from build123d import *

# Parameters (mm, degrees)
SKETCH1_R           = 60.625
SKETCH1_R_2         = 45
BOSS_EXTRUDE1_DEPTH = 4
SKETCH2_R           = 49
SKETCH2_R_2         = 45
BOSS_EXTRUDE2_DEPTH = 52
SKETCH3_W           = 8
SKETCH3_H           = 38
SKETCH3_W_2         = 15
SKETCH3_H_2         = 8
BOSS_EXTRUDE3_DEPTH = 13
SKETCH4_R           = 1.3
CUT_EXTRUDE1_DEPTH  = 7.2
BOSS_EXTRUDE4_DEPTH = 4
SKETCH7_W           = 10
SKETCH7_H           = 24
CUT_EXTRUDE2_DEPTH  = 8
SKETCH8_R           = 5
CUT_EXTRUDE3_DEPTH  = 110.441337026
CUT_EXTRUDE4_REACH  = 104.405
SKETCH9_R           = 1.5


with BuildPart() as part:
    # Sketch1 → Boss-Extrude1 (new body)
    with BuildSketch(Plane(origin=(0, 0, 0), x_dir=(1, 0, 0), z_dir=(0, 1, 0))):
        with Locations(Location((0, 0, 0), (0, 0, 270))):
            Circle(SKETCH1_R)
        with Locations(Location((0, 0, 0), (0, 0, 270))):
            Circle(SKETCH1_R_2, mode=Mode.SUBTRACT)
    extrude(amount=BOSS_EXTRUDE1_DEPTH)

    # Sketch2 → Boss-Extrude2 (add)
    with BuildSketch(Plane(origin=(0, 4, 0), x_dir=(1, 0, 0), z_dir=(0, 1, 0))):
        with Locations(Location((0, 0, 0), (0, 0, 90))):
            Circle(SKETCH2_R)
        with Locations(Location((0, 0, 0), (0, 0, 270))):
            Circle(SKETCH2_R_2, mode=Mode.SUBTRACT)
    extrude(amount=BOSS_EXTRUDE2_DEPTH)

    # Sketch3 → Boss-Extrude3 (add, symmetric)
    with BuildSketch(Plane.XY):
        with Locations((15.25, 19)):
            Rectangle(SKETCH3_W, SKETCH3_H)
        with Locations((-39.25, 34)):
            Rectangle(SKETCH3_W_2, SKETCH3_H_2)
    extrude(amount=BOSS_EXTRUDE3_DEPTH, both=True)


with BuildPart() as boss_extrude3_piece_1:
    # of the separate pieces the step leaves, piece 1, a body of its own (boss_extrude3_pieces)
    add(part.part.solids().sort_by_distance((0, 0, 60.625))[0])


with BuildPart() as boss_extrude3_piece_2:
    # of the separate pieces the step leaves, piece 2, a body of its own (boss_extrude3_pieces)
    add(part.part.solids().sort_by_distance((11.25, 0, -13))[0])


with BuildPart() as cut_extrude1_tool:
    # Sketch4 → Cut-Extrude1 (new body)
    with BuildSketch(Plane(origin=(0, 38, 0), x_dir=(1, 0, 0), z_dir=(0, 1, 0))):
        with Locations(Location((13.75, 5, 0), (0, 0, 270))):
            Circle(SKETCH4_R)
        with Locations(Location((13.75, -5, 0), (0, 0, 270))):
            Circle(SKETCH4_R)
        with Locations(Location((-34.25, 5, 0), (0, 0, 270))):
            Circle(SKETCH4_R)
        with Locations(Location((-34.25, -5, 0), (0, 0, 270))):
            Circle(SKETCH4_R)
    extrude(amount=-CUT_EXTRUDE1_DEPTH)


with BuildPart() as boss_extrude3_piece_1_1:
    add(boss_extrude3_piece_1.part)

    # Cut-Extrude1: cut by cut_extrude1_tool
    add(cut_extrude1_tool.part, mode=Mode.SUBTRACT)



with BuildPart() as boss_extrude3_piece_2_1:
    add(boss_extrude3_piece_2.part)

    # Cut-Extrude1: cut by cut_extrude1_tool
    add(cut_extrude1_tool.part, mode=Mode.SUBTRACT)


with BuildPart() as boss_extrude3_piece_1_2:
    add(boss_extrude3_piece_1_1.part)

    add(boss_extrude3_piece_2_1.part)  # Boss-Extrude4 merges Boss-Extrude3 piece 2
    # Sketch5 → Boss-Extrude4 (add)
    with BuildSketch(Plane.XZ):
        with BuildLine():
            Line((11.25, 13), (25.249838503, 37.248431585))
            ThreePointArc((25.249838503, 37.248431585), (45, 0), (25.249838503, -37.248431585))
            Line((25.249838503, -37.248431585), (11.25, -13))
            Line((11.25, -13), (11.25, 13))
        make_face()
        with BuildLine():
            Line((24.25, -19.516660498), (27.361802413, -24.906460381))
            ThreePointArc((27.361802413, -24.906460381), (37, 0), (27.361802413, 24.906460381))
            Line((27.361802413, 24.906460381), (24.25, 19.516660498))
            Line((24.25, 19.516660498), (24.25, -19.516660498))
        make_face(mode=Mode.SUBTRACT)
    extrude(amount=-BOSS_EXTRUDE4_DEPTH)

    # Sketch7 → Cut-Extrude2 (cut)
    with BuildSketch(Plane.ZY.offset(-11.25)):
        with Locations((0, 17)):
            Rectangle(SKETCH7_W, SKETCH7_H)
    extrude(amount=-CUT_EXTRUDE2_DEPTH, mode=Mode.SUBTRACT)

    # Sketch8 → Cut-Extrude3 (cut, through all)
    with BuildSketch(Plane.ZY.offset(-11.25)):
        with Locations((0, 14)):
            Circle(SKETCH8_R)
    extrude(amount=-CUT_EXTRUDE3_DEPTH, mode=Mode.SUBTRACT)

    # Sketch9 → Cut-Extrude4 (cut, up to next)
    with BuildSketch(Plane.XZ, mode=Mode.PRIVATE) as cut_extrude4_sk1:
        with Locations(Location((54.5, 0, 0), (0, 0, 270))):
            Circle(SKETCH9_R)
    cut_extrude4_tool1 = extrude(cut_extrude4_sk1.sketch, amount=-CUT_EXTRUDE4_REACH, mode=Mode.PRIVATE) & boss_extrude3_piece_1_2.part
    # Sketch9 → Cut-Extrude4 (cut, up to next)
    with BuildSketch(Plane.XZ, mode=Mode.PRIVATE) as cut_extrude4_sk2:
        with Locations(Location((0, -54.5, 0), (0, 0, 270))):
            Circle(SKETCH9_R)
    cut_extrude4_tool2 = extrude(cut_extrude4_sk2.sketch, amount=-CUT_EXTRUDE4_REACH, mode=Mode.PRIVATE) & boss_extrude3_piece_1_2.part
    # Sketch9 → Cut-Extrude4 (cut, up to next)
    with BuildSketch(Plane.XZ, mode=Mode.PRIVATE) as cut_extrude4_sk3:
        with Locations(Location((-54.5, 0, 0), (0, 0, 270))):
            Circle(SKETCH9_R)
    cut_extrude4_tool3 = extrude(cut_extrude4_sk3.sketch, amount=-CUT_EXTRUDE4_REACH, mode=Mode.PRIVATE) & boss_extrude3_piece_1_2.part
    # Sketch9 → Cut-Extrude4 (cut, up to next)
    with BuildSketch(Plane.XZ, mode=Mode.PRIVATE) as cut_extrude4_sk4:
        with Locations(Location((0, 54.5, 0), (0, 0, 270))):
            Circle(SKETCH9_R)
    cut_extrude4_tool4 = extrude(cut_extrude4_sk4.sketch, amount=-CUT_EXTRUDE4_REACH, mode=Mode.PRIVATE) & boss_extrude3_piece_1_2.part
    add(cut_extrude4_tool1.solids().sort_by_distance((54.5, 0, 0))[0], mode=Mode.SUBTRACT)
    add(cut_extrude4_tool2.solids().sort_by_distance((0, 0, -54.5))[0], mode=Mode.SUBTRACT)
    add(cut_extrude4_tool3.solids().sort_by_distance((-54.5, 0, 0))[0], mode=Mode.SUBTRACT)
    add(cut_extrude4_tool4.solids().sort_by_distance((0, 0, 54.5))[0], mode=Mode.SUBTRACT)


solid = boss_extrude3_piece_1_2.part
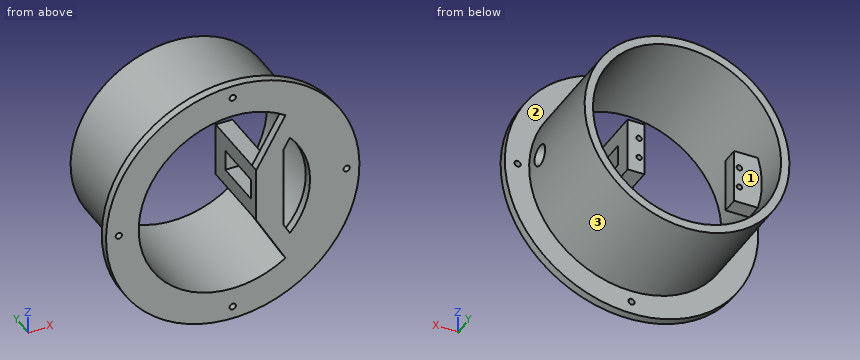
Here's how the part is built. I have some questions about the finished solid (model axes, mm). Face numbers are marked on the shaded views. Give positions to 0.01 mm unless a question says otherwise; leave off trailing zeros. Loops run counter-clockwise (first coordinate to the right, second up) from the corner with the lowest first, then second, coordinate; pieces in that order, holes last. Notation, with made-up numbers: (87.25, 24) -> (134.25, 24) arc R6 cw to (134.25, 30) -> close; hole circle Ø11 at (44.5, 13.25). An arc over 180 degrees is marked (long way). Answer as a JSON object with one key per item and string values. Group by question number.
Item 1: Imagine slicing it at B-B on x = 0. Write out the boundary of the cut face in (y, z) (3 decimals), then the cut area to 3 significant figures.
Item 2: I need wall thicknesses on L1, parallel to X at y = 29.5, z = -11.5; L2, parallel to X at y = 43, z = 0; L3, parallel to Y at x = 45.85, z = 0. Which ranges of each line are inside material? Lowest first, please.
Item 3: Will these pins go through, and if not, where does the flat tip stop? pin 1 (6.5 mm diameter, centred on x = 14, z = 1, fed in from +Y); pin 2 (2 mm diameter, centred on y = 1, z = -8.5, fed in from +X); pin 3 (6.5 mm diameter, centred on x = -39.5, y = 36, fed in from -Z); pin 4 (12 mm diameter, centred on x = 20, z = -14.5, fed in from -Y).
Item 4: Imagine slicing it at A-A on y = 26. Write out the boundary of the cut face in (x, z), then the cut area to 3 significant figures.
Item 5: Thinking about a two-plate mould opening in X: for the marked faces 1, 2 and 3, which applies, pulls with the +X half, pulls with the -X half, needs draft (parallel to the pull), parting line crosses it, or undercut?
Item 6: Imagine slicing it at C-C on z = 39.5. Write out the boundary of the cut face in (x, y), then the cut area to 3 significant figures.
Item 7: Imagine slicing it at D-D on x = 54.5. Write out the boundary of the cut face in (y, z).
Answer list:
{
 "1": {"outline": "(0, -60.625) -> (4, -60.625) -> (4, -56) -> (0, -56) -> close; (0, -53) -> (4, -53) -> (4, -49) -> (56, -49) -> (56, -45) -> (0, -45) -> close; (0, 45) -> (56, 45) -> (56, 49) -> (4, 49) -> (4, 53) -> (0, 53) -> close; (0, 56) -> (4, 56) -> (4, 60.625) -> (0, 60.625) -> close", "area": "517 mm2"},
 "2": {"L1": "x = -47.63 to -43.51, 11.25 to 19.25, 43.51 to 47.63", "L2": "x = -49 to -45, 45 to 49", "L3": "y = 0 to 9, 19 to 56"},
 "3": {"pin 1": "stops at y = 38", "pin 2": "stops at x = 60.16", "pin 3": "stops at z = -32.97", "pin 4": "stops at y = 0"},
 "4": {"outline": "circle Ø98 at (0, 0); (11.25, -13) -> (19.25, -13) -> (19.25, -5) -> (11.25, -5) -> close; (11.25, 5) -> (19.25, 5) -> (19.25, 13) -> (11.25, 13) -> close; hole circle Ø90 at (0, 0)", "area": "1,310 mm2"},
 "5": {"face 1": "undercut", "face 2": "needs draft", "face 3": "parting line crosses it"},
 "6": {"outline": "(-45.99, 0) -> (-21.56, 0) -> (-21.56, 56) -> (-29, 56) -> (-29, 4) -> (-45.99, 4) -> close; (21.56, 0) -> (45.99, 0) -> (45.99, 4) -> (29, 4) -> (29, 56) -> (21.56, 56) -> close", "area": "969 mm2"},
 "7": {"outline": "(0, -26.55) -> (4, -26.55) -> (4, -1.5) -> (0, -1.5) -> close; (0, 1.5) -> (4, 1.5) -> (4, 26.55) -> (0, 26.55) -> close"}
}
